Design review of the part shown in the three views and the two pictorial views. Dimensions are in mm from the part's minimum x, y and z. A direction names the side the tool comes from. Round coordinates to 2 decimals unless told otherwise and drop trailing zeros. Loops run counter-clockwise (first coordinate to the right, second up) from the corner with the lowest first, then second, coordinate; pieces in that order, holes last. Notation, with made-up numbers: (40.25, 35) -> (63.25, 35) arc R7 ccw to (63.25, 41) -> close; hole circle Ø1 at (8, 11). An arc over 180 degrees is marked (long way). Return JSON: item names as keys, results as strings. Group by question number.
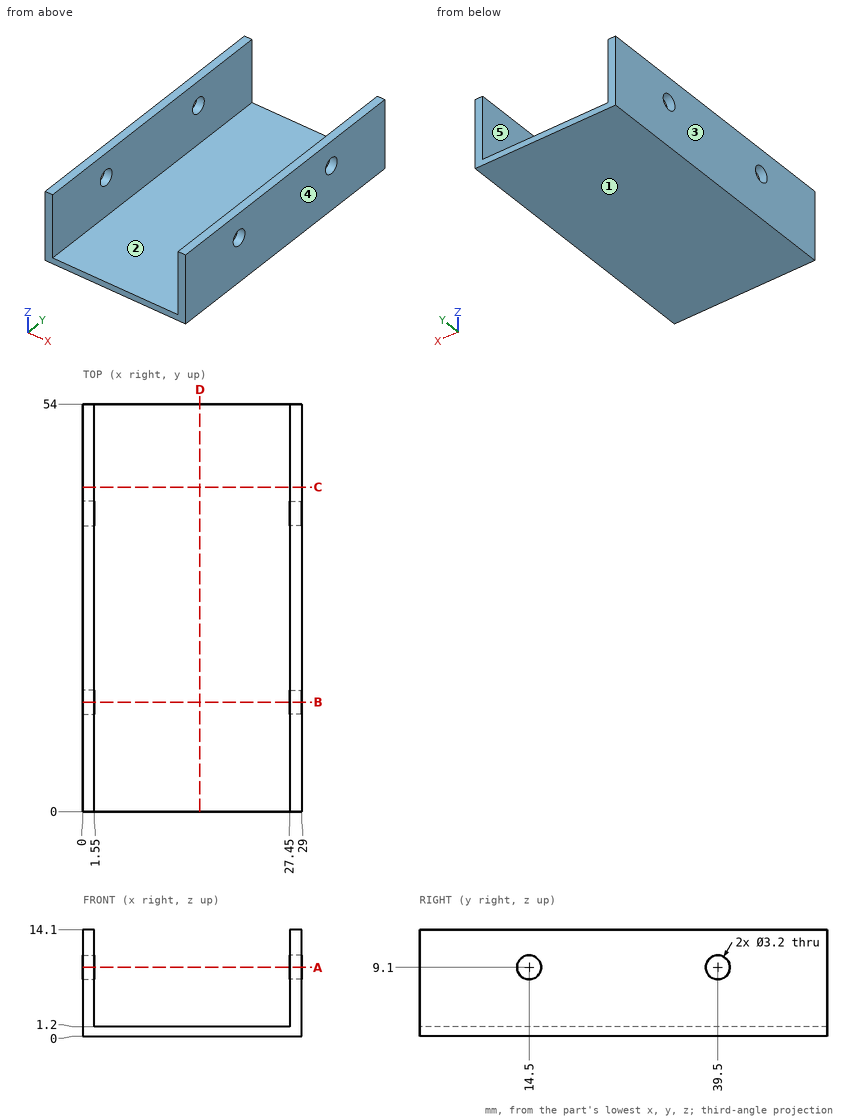
1. Draft analysis for pull direction X (two halves, no side actions). For the marked faces 3, 4 and 5, state which applies: pulls with the +X half, pulls with the -X half, needs draft (parallel to the pull), parting line crosses it, or undercut.
2. We need section B-B, the plane y = 14.5. Write out the cut boundary in (x, z).
3. We need section D-D, the plane x = 15.5. Write out the cut boundary in (y, z), then the cut area to 3 significant figures.
4. Wall thickness on line 1 (Y direction, x = 28, z = 9.1); line 2 (X direction, y = 28.5, z = 3); line 3 (Z direction, x = 0.8, y = 14.5): over which ranges is each line inside the solid? List them lowest first.
5. We need section C-C, the plane y = 43. Write out the cut boundary in (x, z), then the cut area to 3 significant figures.
6. For P1, Ø4, axis at x = 12, y = 17, coming from the +Z side; P2, Ø3, axis at y = 14.5, z = 9.1, coming from the -X side, all flat-tipped, find the tip position at first contact; note any pin that passes through.
7. Tool access review of the marked faces 1 and 2: name each direction out of +Z, -Z, +X, -X, +Y, -Y from which nothing blocks a thin tool from reaching the whole face with its end or side.
8. We need section A-A, the plane z = 9.1. Write out the cut boundary in (x, y).
Check sheet entries:
{
 "1": {"face 3": "pulls with the -X half", "face 4": "pulls with the +X half", "face 5": "undercut"},
 "2": {"outline": "(0, 0) -> (29, 0) -> (29, 7.5) -> (27.45, 7.5) -> (27.45, 1.2) -> (1.55, 1.2) -> (1.55, 7.5) -> (0, 7.5) -> close; (0, 10.7) -> (1.55, 10.7) -> (1.55, 14.1) -> (0, 14.1) -> close; (27.45, 10.7) -> (29, 10.7) -> (29, 14.1) -> (27.45, 14.1) -> close"},
 "3": {"outline": "(0, 0) -> (54, 0) -> (54, 1.2) -> (0, 1.2) -> close", "area": "64.8 mm²"},
 "4": {"line 1": "y = 0 to 12.9, 16.1 to 37.9, 41.1 to 54", "line 2": "x = 0 to 1.55, 27.45 to 29", "line 3": "z = 0 to 7.5, 10.7 to 14.1"},
 "5": {"outline": "(0, 0) -> (29, 0) -> (29, 14.1) -> (27.45, 14.1) -> (27.45, 1.2) -> (1.55, 1.2) -> (1.55, 14.1) -> (0, 14.1) -> close", "area": "74.8 mm²"},
 "6": {"P1": "stops at z = 1.2", "P2": "passes through"},
 "7": {"face 1": "-Z, +X, -X, +Y, -Y", "face 2": "+Z, +Y, -Y"},
 "8": {"outline": "(0, 0) -> (1.55, 0) -> (1.55, 12.9) -> (0, 12.9) -> close; (0, 16.1) -> (1.55, 16.1) -> (1.55, 37.9) -> (0, 37.9) -> close; (0, 41.1) -> (1.55, 41.1) -> (1.55, 54) -> (0, 54) -> close; (27.45, 0) -> (29, 0) -> (29, 12.9) -> (27.45, 12.9) -> close; (27.45, 16.1) -> (29, 16.1) -> (29, 37.9) -> (27.45, 37.9) -> close; (27.45, 41.1) -> (29, 41.1) -> (29, 54) -> (27.45, 54) -> close"}
}
